```python
from build123d import *

# Parameters (mm, degrees)
ESQUISSE1_R                  = 34
BOSS_EXTRU_1_DEPTH           = 2
ESQUISSE2_R                  = 36.5
ESQUISSE2_R_2                = 34
BOSS_EXTRU_2_DEPTH           = 15
BOSS_EXTRU_2_DEPTH_BACK      = 2
ESQUISSE3_R                  = 4.05
ENL_V_MAT_EXTRU_1_DEPTH      = 16
ENL_V_MAT_EXTRU_1_DEPTH_BACK = 3


with BuildPart() as part:
    # Esquisse1 → Boss.-Extru.1 (new body)
    with BuildSketch(Plane.XY):
        Circle(ESQUISSE1_R)
    extrude(amount=BOSS_EXTRU_1_DEPTH)

    # Esquisse2 → Boss.-Extru.2 (add, two sides)
    with BuildSketch(Plane.XY.offset(2)) as boss_extru_2_sk:
        Circle(ESQUISSE2_R)
        Circle(ESQUISSE2_R_2, mode=Mode.SUBTRACT)
    extrude(amount=BOSS_EXTRU_2_DEPTH)
    extrude(boss_extru_2_sk.sketch, amount=-BOSS_EXTRU_2_DEPTH_BACK)

    # Esquisse3 → Enlèv. mat.-Extru.1 (cut, two sides)
    with BuildSketch(Plane.XY.offset(2)) as enl_v_mat_extru_1_sk:
        Circle(ESQUISSE3_R)
    extrude(amount=ENL_V_MAT_EXTRU_1_DEPTH, mode=Mode.SUBTRACT)
    extrude(enl_v_mat_extru_1_sk.sketch, amount=-ENL_V_MAT_EXTRU_1_DEPTH_BACK, mode=Mode.SUBTRACT)


solid = part.part
```
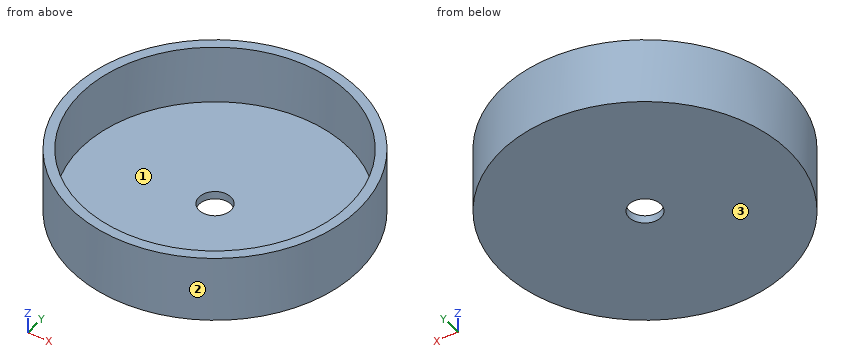
Geometry check sheet. Reference: the model listing, model coordinates, mm. Face numbers are marked on the shaded views. Coordinates: 2 decimals unless noted, no trailing zeros. Write each loop counter-clockwise with the first axis right and the second up, starting at its lowest first coordinate (ties: lowest second). Pieces come first, ordered by that corner, then holes. Notation, with made-up numbers: (-8, 78) -> (30, 78) arc R3 cw to (30, 82) -> close; hole circle Ø8 at (44, -21.5). An arc over 180 degrees is marked (long way). Use CSV: the item, a comma, the result in double quotes. Start each with the question number.
Item 1: Cross-section at A-A, the plane y = 0. Record the cut outline in (x, z), plus the area to 3 significant figures.
Item 2: Thickness scan on line 1 (Y direction, x = 0, z = 1.15); line 2 (Y direction, x = 0, z = 7); line 3 (X direction, y = -21.5, z = 11). Record the ranges inside material, lowest first.
Item 3: Cross-section at C-C, the plane z = 14.5. Record the cut outline in (x, y).
Item 4: Mould release check, pull along Y, two halves, no side actions. Record for the marked faces 1, 2 and 3: released by +Y, released by -Y, zero draft, split by the parting line, or undercut.
Item 5: Cross-section at D-D, the plane x = -13. Record the cut outline in (y, z), plus the area to 3 significant figures.
Item 6: Depth check by flat-ended pin: pin 1 Ø3 at (y, z) = (-10.5, 6.5) entering from -X; pin 2 Ø1.5 at (y, z) = (-9.5, 10) entering from +X; pin 3 Ø10 at (x, y) = (-5, 7) entering from +Z. Enter the tip coordinate at first touch or a pass-through.
Answers:
1,outline,"(-36.5, 0) -> (-4.05, 0) -> (-4.05, 2) -> (-34, 2) -> (-34, 17) -> (-36.5, 17) -> close; (4.05, 0) -> (36.5, 0) -> (36.5, 17) -> (34, 17) -> (34, 2) -> (4.05, 2) -> close"
1,area,"205 mm^2"
2,line 1,"-36.5 to -4.05, 4.05 to 36.5"
2,line 2,"-36.5 to -34, 34 to 36.5"
2,line 3,"-29.5 to -26.34, 26.34 to 29.5"
3,outline,"circle Ø73 at (0, 0); hole circle Ø68 at (0, 0)"
4,face 1,"undercut"
4,face 2,"split by the parting line"
4,face 3,"zero draft"
5,outline,"(-34.11, 0) -> (34.11, 0) -> (34.11, 17) -> (31.42, 17) -> (31.42, 2) -> (-31.42, 2) -> (-31.42, 17) -> (-34.11, 17) -> close"
5,area,"217 mm^2"
6,pin 1,"x = -35.37"
6,pin 2,"x = 35.44"
6,pin 3,"z = 2"
